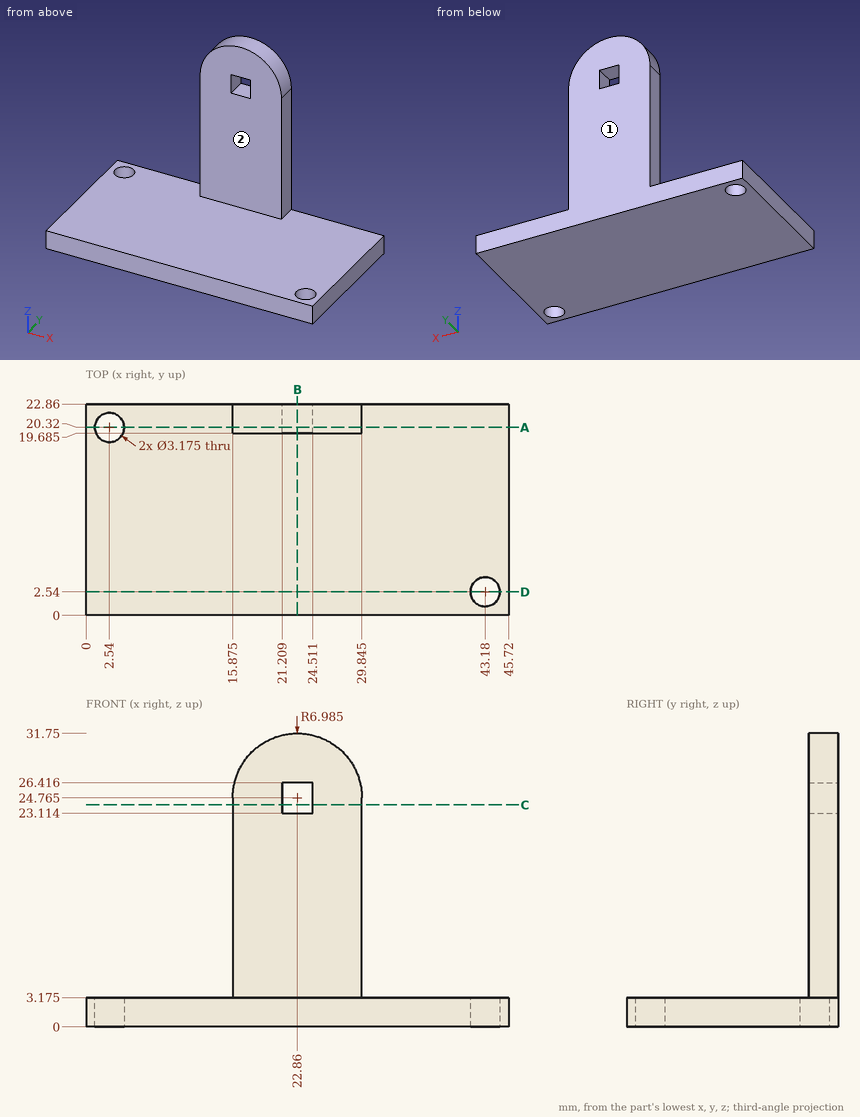
Study the drawing (mm; zero at the part's minimum x, y, z) and answer. A direction names the side the tool comes from. Round coordinates to 2 decimals unless told otherwise and drop trailing zeros. Loops run counter-clockwise (first coordinate to the right, second up) from the corner with the lowest first, then second, coordinate; pieces in that order, holes last. Notation, with made-up numbers: (-4.5, 56) - (50.5, 56) arc R20 cw to (50.5, 80) - close; hole circle Ø8 at (-40, -19). An arc over 180 degrees is marked (long way). Use one line per item in the form item = value. Start each with the question number.
1. Consider line 1 (Y direction, x = 43, z = 1); line 2 (X direction, y = 2.54, z = 1.5); line 3 (X direction, y = 20.32, z = 0.6). Determine where each line is inside the solid, lowest interval first. Write a range as [from, to].
2. The part is cut by section D-D on y = 2.54. Determine the outline of the cut face in (x, z) (1 decimal).
3. Given pin 1 Ø1.6 at (y, z) = (21, 24) entering from -X (3 decimals); pin 2 Ø1 at (x, z) = (21, 20.5) entering from -Y (3 decimals); pin 3 Ø2.5 at (y, z) = (21, 13) entering from +X (3 decimals); pin 4 Ø2.5 at (x, y) = (43.18, 2.54) entering from +Z, each flat-ended and moving along its own axis, determine where each tip first touches the part or whether it passes through.
4. The part is cut by section C-C on z = 24. Determine the outline of the cut face in (x, y) (3 decimals).
5. A tool of negligible diameter and unlimited length cuts with its end or side. For the marked faces 1 and 2, from which of +Z, -Z, +X, -X, +Y, -Y can it reach the whole face along a straight path? Write none if from no direction.
6. The part is cut by section A-A on y = 20.32. Determine the outline of the cut face in (x, z) (1 decimal), then the cut area to 3 significant figures.
7. The part is cut by section B-B on x = 22.86. Determine the outline of the cut face in (y, z) (3 decimals).
Geometry check:
q1.line_1 = [0, 0.96], [4.12, 22.86]
q1.line_2 = [0, 41.59], [44.77, 45.72]
q1.line_3 = [0, 0.95], [4.13, 45.72]
q2.outline = (0, 0) - (41.6, 0) - (41.6, 3.2) - (0, 3.2) - close; (44.8, 0) - (45.7, 0) - (45.7, 3.2) - (44.8, 3.2) - close
q3.pin_1 = 15.875
q3.pin_2 = 19.685
q3.pin_3 = 29.845
q3.pin_4 = through
q4.outline = (15.875, 19.685) - (21.209, 19.685) - (21.209, 22.86) - (15.875, 22.86) - close; (24.511, 19.685) - (29.845, 19.685) - (29.845, 22.86) - (24.511, 22.86) - close
q5.face_1 = +Z, -Z, +X, -X, +Y
q5.face_2 = +Z, +X, -X, -Y
q6.outline = (0, 0) - (1, 0) - (1, 3.2) - (0, 3.2) - close; (4.1, 0) - (45.7, 0) - (45.7, 3.2) - (29.8, 3.2) - (29.8, 24.8) arc R7 ccw to (15.9, 24.8) - (15.9, 3.2) - (4.1, 3.2) - close; hole (21.2, 23.1) - (24.5, 23.1) - (24.5, 26.4) - (21.2, 26.4) - close
q6.area = 502 mm^2
q7.outline = (0, 0) - (22.86, 0) - (22.86, 23.114) - (19.685, 23.114) - (19.685, 3.175) - (0, 3.175) - close; (19.685, 26.416) - (22.86, 26.416) - (22.86, 31.75) - (19.685, 31.75) - close
